Could you check a few things on this drawing? It's one solid part, dimensions in mm from its lowest x, y, z. Round coordinates to 2 decimals unless told otherwise and drop trailing zeros. Write each loop counter-clockwise with the first axis right and the second up, starting at its lowest first coordinate (ties: lowest second). Pieces come first, ordered by that corner, then holes. Notation, with made-up numbers: (63.5, -14.5) -> (104.5, -14.5) arc R19 cw to (104.5, -3.5) -> close; hole circle Ø3 at (-19, 16.5). An arc over 180 degrees is marked (long way). Return JSON: item names as keys, results as strings.
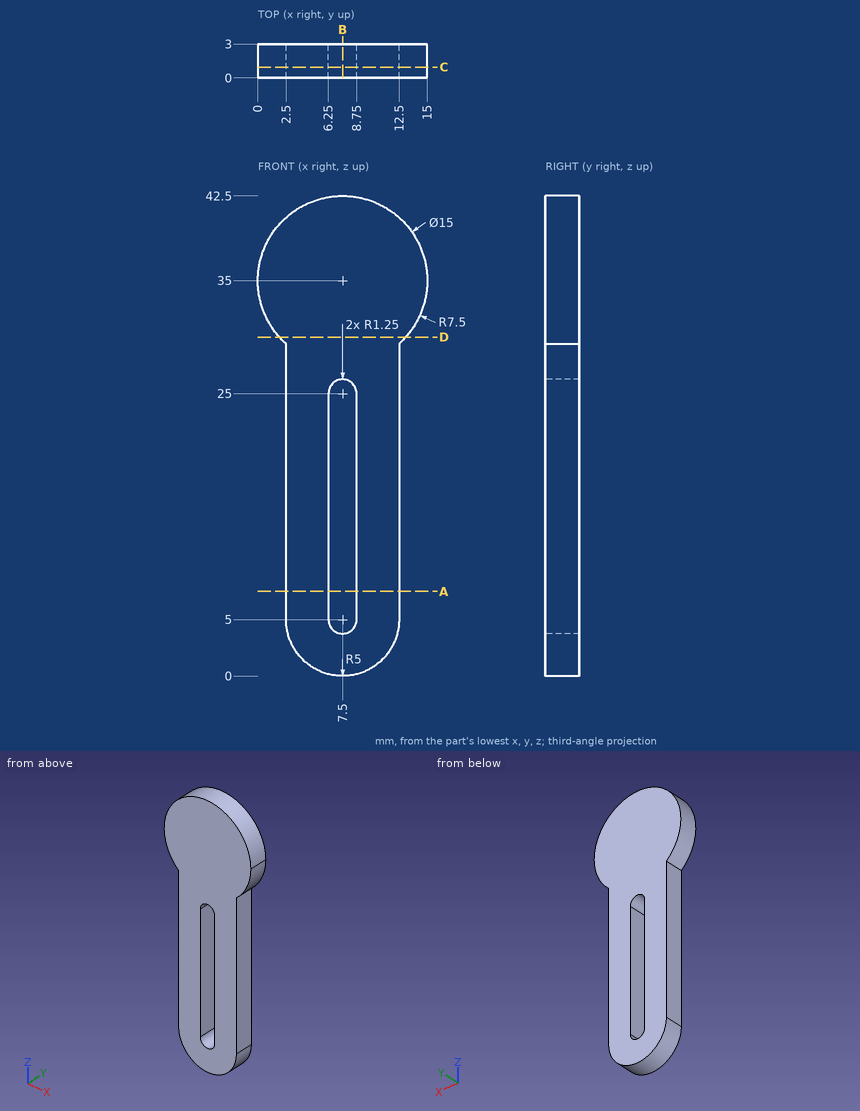
1) Will these pins go through, and if not, where does the flat tip stop? pin 1 Ø1.5 at (x, y) = (10.5, 1) entering from +Z; pin 2 Ø0.9 at (y, z) = (2, 15) entering from +X.
Return value:
{"pin 1": "z = 42.15", "pin 2": "x = 12.5"}
2) I want a section at B-B, the plane x = 7.5. Please give me the cut outline in (y, z).
Return value:
{"outline": "(0, 0) -> (3, 0) -> (3, 3.75) -> (0, 3.75) -> close; (0, 26.25) -> (3, 26.25) -> (3, 42.5) -> (0, 42.5) -> close"}
3) If I drill on probe 1 along X at (y, z) = (0.2, 6); probe 2 along X at (y, z) = (0.6, 26.5); probe 3 along X at (y, z) = (0.5, 4.5), over which ranges is the centre line in solid material (lowest first)? Write a range as [from, to].
Return value:
{"probe 1": "[2.5, 6.25], [8.75, 12.5]", "probe 2": "[2.5, 12.5]", "probe 3": "[2.53, 6.35], [8.65, 12.47]"}
4) I want a section at C-C, the plane y = 0.95. Please give me the cut outline in (x, z).
Return value:
{"outline": "(2.5, 5) arc R5 ccw to (12.5, 5) -> (12.5, 29.41) arc R7.5 ccw (long way) to (2.5, 29.41) -> close; hole (6.25, 5) arc R1.25 ccw to (8.75, 5) -> (8.75, 25) arc R1.25 ccw to (6.25, 25) -> close"}
5) I want a section at A-A, the plane z = 7.5. Please give me the cut outline in (x, y).
Return value:
{"outline": "(2.5, 0) -> (6.25, 0) -> (6.25, 3) -> (2.5, 3) -> close; (8.75, 0) -> (12.5, 0) -> (12.5, 3) -> (8.75, 3) -> close"}
6) I want a section at D-D, the plane z = 30. Please give me the cut outline in (x, y), and give its area (3 significant figures).
Return value:
{"outline": "(1.91, 0) -> (13.09, 0) -> (13.09, 3) -> (1.91, 3) -> close", "area": "33.5 mm²"}
